Autodesk Inventor part; units mm, degrees
ref_plane "YZ Plane" through (0, 0, 0) normal (1, 0, 0) x (0, 1, 0)
ref_plane "XZ Plane" through (0, 0, 0) normal (0, 1, 0) x (-1, 0, 0)
ref_plane "XY Plane" through (0, 0, 0) normal (0, 0, 1) x (1, 0, 0)
sketch "Sketch1" plane through (0, 0, 0) normal (0, 0, 1) x (1, 0, 0)
  line L0 (7.3, 7.5) -> (0.2, 7.5)
  line L1 (0, 7.3) -> (0, 0.2)
  line L2 (0.2, 0) -> (7.3, 0)
  line L3 (7.5, 0.2) -> (7.5, 7.3)
  arc A0 (7.5, 7.3) -> (7.3, 7.5) centre (7.3, 7.3) ccw
  arc A1 (0.2, 7.5) -> (0, 7.3) centre (0.2, 7.3) ccw
  arc A2 (0, 0.2) -> (0.2, 0) centre (0.2, 0.2) ccw
  arc A3 (7.3, 0) -> (7.5, 0.2) centre (7.3, 0.2) ccw
  point P0 (0, 0)
  point P1 (0, 7.5)
  point P2 (7.5, 0)
  dimension "d0" = 7.5
  dimension "d1" = 7.5
  dimension "d2" = 0.2
extrude "Extrusion1" add sketch "Sketch1" along normal mid plane 3
sketch "Sketch3" plane through (0, 0, 0) normal (0, 0, 1) x (1, 0, 0)
  line L0 (0, 7.3) -> (0, 0.2)
  line L1 (1.4869, 3.75) -> (1.4869, 1.25)
  line L2 (1.4869, 1.25) -> (5.2369, 1.25)
  line L3 (1.4869, 3.75) -> (1.4869, 6.25)
  line L4 (1.4869, 6.25) -> (5.2369, 6.25)
  line L5 (1.4869, 1.25) -> (0, 1.25)
  line L6 (0, 1.25) -> (3.75, 1.25)
  line L7 (3.75, 1.25) -> (3.75, 6.25)
  line L8 (3.75, 6.25) -> (0, 6.25)
  point P0 (0, 0)
  dimension "d7" = 2.5
  dimension "d8" = 3.75
  dimension "d9" = 2.5
  dimension "d10" = 3.75
  dimension "d11" = 3.75
  dimension "d12" = 5
  dimension "d13" = 3.75
ref_plane "Work Plane1" through (3.75, 0.2, 1.5) normal (-1, 0, 0) x (0, 0, 1)
sketch "Sketch4" plane through (3.75, 0.2, 1.5) normal (-1, 0, 0) x (0, 0, 1)
  line L0 (-1.5, 6.4485) -> (23.5, 6.4485)
  line L1 (-1.5, 0.671) -> (23.5, 0.671)
  point P0 (-1.5, -0.2)
  dimension "d15" = 25
  dimension "d17" = 25
ref_plane "Work Plane2" through (0, 0, 1.5) normal (0, 0, 1) x (1, 0, 0)
sketch "Sketch6" plane through (0, 0, 1.5) normal (0, 0, 1) x (1, 0, 0)
  circle A0 centre (3.7506, 6.6485) radius 0.35
  circle A1 centre (3.7506, 0.8713) radius 0.35
  point P0 (0, 0)
  dimension "d22" = 0.7
  dimension "d27" = 0.7
extrude "Extrusion3" add sketch "Sketch6" along normal blind 0.5 contours A0
fillet "Fillet3" radius 0.2 2 edges at (3.4006, 6.6485, 1.5) (3.4006, 6.6485, 2)
extrude "Extrusion4" add sketch "Sketch6" along normal blind 0.5 contours A1
fillet "Fillet4" radius 0.2 2 edges at (3.4006, 0.8713, 2) (3.4006, 0.8713, 1.5)
ref_plane "Work Plane3" through (3.7506, 0.8713, 2) normal (0, 0, 1) x (1, 0, 0)
ref_plane "Work Plane4" through (3.7506, 6.6485, 2) normal (0, 0, 1) x (1, 0, 0)
sketch "Sketch7" plane through (3.7506, 0.8713, 2) normal (0, 0, 1) x (1, 0, 0)
  circle A0 centre (0, 0) radius 0.25
  point P0 (-3.7506, -0.8713)
  dimension "d33" = 0.5
sweep "Sweep1" add profiles "Sketch7" path "Sketch4" path curves L1
sketch "Sketch8" plane through (3.7506, 6.6485, 2) normal (0, 0, 1) x (1, 0, 0)
  circle A0 centre (0, 0) radius 0.25
  point P0 (-3.7506, -6.6485)
  dimension "d36" = 0.5
sweep "Sweep2" add profiles "Sketch8" path "Sketch4" path curves L0
equation "\"BendRadius\" = Thickness"
equation "\"BendReliefWidth\" = Thickness"
equation "\"BendReliefDepth\" = 0.5 * Thickness"
equation "\"CornerReliefSize\" = 4 * Thickness"
equation "\"MinimumRemnant\" = 2 * Thickness"
equation "\"TransitionRadius\" = BendRadius"
equation "\"JacobiRadiusSize\" = BendRadius"
equation "\"GapSize\" = Thickness"
properties part number "A60"
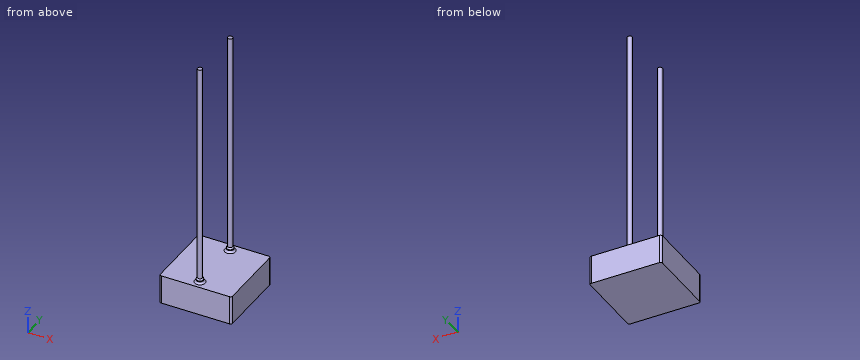
Read the model definition and answer for the solid it produces. Units are mm, in the model's axes. Round coordinates to 2 decimals unless told otherwise and drop trailing zeros. Write each loop counter-clockwise with the first axis right and the second up, starting at its lowest first coordinate (ties: lowest second). Pieces come first, ordered by that corner, then holes. Notation, with made-up numbers: M 14.5,76 L 18.5,76 A21 cw 18.5,113 Z; hole C -17.75,-26 d2. An arc over 180 degrees is marked long. One line per item, written item: value.
Q1. Find section B-B on z = 22. Write down the section's boundary in (x, y), plus the area to 3 significant figures.
Data:
outline: C 3.75,0.87 d0.5; C 3.75,6.65 d0.5
area: 0.393 mm2
Q2. Straight lines are drawn through the part: line 1 (Y direction, x = 3.75, z = 2.5); line 2 (Z direction, x = 2.5, y = 6.5). For each, find the intervals that lie inside material, in ascending order. Write a range as [from, to].
Data:
line 1: [0.62, 1.12], [6.4, 6.9]
line 2: [-1.5, 1.5]
Q3. Flat-ended cylindrical pins translate along their axes: pin 1 Ø1 at (x, y) = (3, 5) entering from +Z; pin 2 Ø1 at (y, z) = (5.5, 12.5) entering from -X. Find the tip coordinate at first contact, or state that the pin passes through.
Data:
pin 1: z = 1.5
pin 2: through
Q4. Find section A-A on y = 1.75. Write down the section's boundary in (x, z), plus the area to 3 significant figures.
Data:
outline: M 0,-1.5 L 7.5,-1.5 L 7.5,1.5 L 0,1.5 Z
area: 22.5 mm2
